Here's the drawing with two shaded views (mm, measured from the low corner). I have some questions. A direction names the side the tool comes from. Give positions to 0.01 mm unless a question says otherwise; leave off trailing zeros. Loops run counter-clockwise (first coordinate to the right, second up) from the corner with the lowest first, then second, coordinate; pieces in that order, holes last.
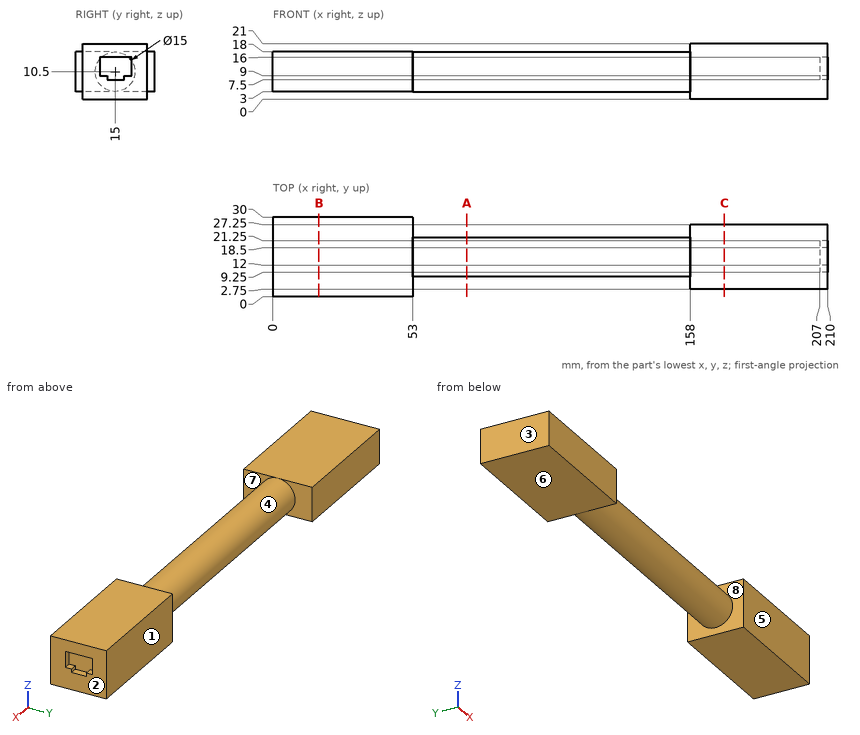
(1) Thinking about a two-plate mould opening in X: for the marked faces 1, 2, 3 and 4, which applies, pulls with the +X half, pulls with the -X half, needs draft (parallel to the pull), parting line crosses it, or undercut?
Returned:
face 1: needs draft
face 2: pulls with the +X half
face 3: pulls with the -X half
face 4: undercut
(2) Which directions (+Z, -Z, +X, -X, +Y, -Y) give clear straight access to the entire face, cutting with the end or side of a thin tool? Please do the marked faces 5, 6, 7 and 8.
Returned:
face 5: +Z, -Z, +X, -Y
face 6: -Z, -X, +Y, -Y
face 7: -Y
face 8: none
(3) Please list where these lines run through material, in increasing order: probe 1 along X at (y, z) = (26, 3.5); probe 2 along Z at (x, y) = (21, 3.5); probe 3 along Y at (x, z) = (177, 14).
Returned:
probe 1: x = 0 to 53, 158 to 210
probe 2: z = 3 to 18
probe 3: y = 2.75 to 27.25
(4) Suppose I cut it at C-C on x = 171. List the corners of the cut face in (y, z) for me, plus the area to 4 significant figures.
Returned:
outline: (2.75, 0) - (27.25, 0) - (27.25, 21) - (2.75, 21) - close
area: 514.5 mm2
(5) Will these pins go through, and if not, where does the flat tip stop? P1, Ø9, axis at x = 15, y = 18, coming from the +Z side; P2, Ø1, axis at x = 70.5, y = 9, coming from the -Z side; P3, Ø1.2, axis at x = 209, z = 8, coming from the -Y side; P4, Ø5, axis at x = 61.5, y = 3.5, coming from the +Z side.
Returned:
P1: stops at z = 18
P2: stops at z = 5.4
P3: stops at y = 2.75
P4: passes through
(6) Suppose I cut it at B-B on x = 17.5. List the corners of the cut face in (y, z) for me, plus the area to 3 significant figures.
Returned:
outline: (0, 3) - (30, 3) - (30, 18) - (0, 18) - close
area: 450 mm2
(7) Suppose I cut it at A-A on x = 73.5. List the corners of the cut face in (y, z) for me.
Returned:
outline: circle Ø15 at (15, 10.5)
